Geometry check sheet. Reference: the model listing, model coordinates, mm. Face numbers are marked on the shaded views. A direction names the side the tool comes from. Coordinates: 2 decimals unless noted, no trailing zeros. Write each loop counter-clockwise with the first axis right and the second up, starting at its lowest first coordinate (ties: lowest second). Pieces come first, ordered by that corner, then holes.
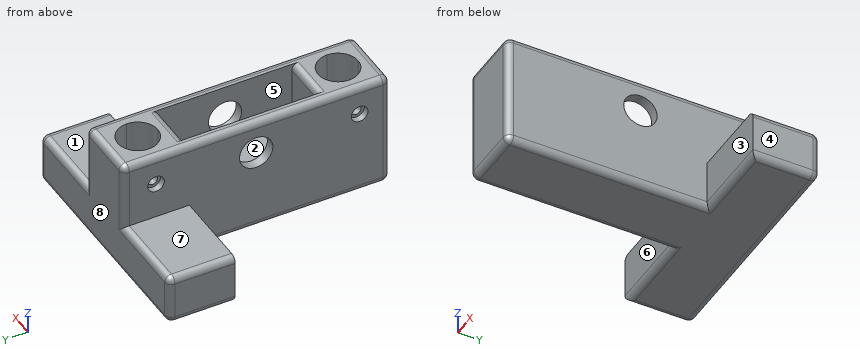
from build123d import *

# Parameters (mm, degrees)
F1_DEPTH        = 15
F2_W            = 20
F2_H            = 20
F3_DEPTH        = 20
F5_DEPTH        = 15
F6_W            = 20
F6_H            = 20
F7_DEPTH        = 20
F9_DEPTH        = 15
F10_W           = 3
F10_H           = 40
F11_DEPTH       = 20
F12_R           = 5
F13_DEPTH       = 25
F14_R           = 2
F15_R           = 2
F16_R           = 2
F17_R           = 2
F19_D           = 3.1
F19_DEPTH       = 6
F19_CBORE_D     = 5
F19_CBORE_DEPTH = 2


with BuildPart() as f1:
    # F0 (on Top) → F1 (new body)
    with BuildSketch(Plane.XY):
        Polygon((-20, 0), (0, 0), (0, 60), (25, 60), (25, 80), (-45, 80), (-45, 60), (-20, 60), align=None)
    extrude(amount=F1_DEPTH)

    # F2 (on face) → F3 (join)
    with BuildSketch(Plane.XY.offset(15)):
        with Locations((-10, 10)):
            Rectangle(F2_W, F2_H)
    extrude(amount=F3_DEPTH)

    # F4 (on face) → F5 (cut)
    with BuildSketch(Plane.XY.offset(35)):
        with BuildLine():
            ThreePointArc((-10, 4), (-5.757359, 5.757359), (-4, 10))
            ThreePointArc((-4, 10), (-14.242641, 14.242641), (-10, 4))
        make_face()
    extrude(amount=-F5_DEPTH, mode=Mode.SUBTRACT)

    # F6 (on face) → F7 (join)
    with BuildSketch(Plane.XY.offset(15)):
        with Locations((-10, 70)):
            Rectangle(F6_W, F6_H)
    extrude(amount=F7_DEPTH)

    # F8 (on face) → F9 (cut)
    with BuildSketch(Plane.XY.offset(35)):
        with BuildLine():
            ThreePointArc((-10, 64), (-5.757359, 65.757359), (-4, 70))
            ThreePointArc((-4, 70), (-14.242641, 74.242641), (-10, 64))
        make_face()
    extrude(amount=-F9_DEPTH, mode=Mode.SUBTRACT)

    # F10 (on face) → F11 (join)
    with BuildSketch(Plane.XY.offset(15)):
        with Locations((-1.5, 40)):
            Rectangle(F10_W, F10_H)
        with Locations((-18.5, 40)):
            Rectangle(F10_W, F10_H)
    extrude(amount=F11_DEPTH)

    # F12 (on face) → F13 (cut)
    with BuildSketch(Plane(origin=(-20, 0, 0), x_dir=(0, -1, 0), z_dir=(-1, 0, 0))):
        with Locations((-40, 25)):
            Circle(F12_R)
    extrude(amount=-F13_DEPTH, mode=Mode.SUBTRACT)

    # F14
    f14_edges = [f1.edges().sort_by_distance(p)[0] for p in [
        (-20, 40, 35),
        (0, 40, 35),
    ]]
    fillet(f14_edges, radius=F14_R)

    # F15
    f15_edges = [f1.edges().sort_by_distance(p)[0] for p in [
        (-10, 20, 35),
        (-10, 60, 35),
        (-10, 80, 35),
        (-10, 0, 35),
    ]]
    fillet(f15_edges, radius=F15_R)

    # F16
    f16_edges = [f1.edges().sort_by_distance(p)[0] for p in [
        (-1, 80, 15),
        (12.5, 80, 15),
        (-19, 80, 15),
        (-32.5, 80, 15),
    ]]
    fillet(f16_edges, radius=F16_R)

    # F17
    f17_edges = [f1.edges().sort_by_distance(p)[0] for p in [
        (-20, 31, 0),
        (-32.5, 60, 0),
        (12.5, 60, 0),
        (-45, 70, 0),
        (25, 70, 0),
        (-10, 80, 0),
        (-45, 80, 6.5),
        (25, 80, 6.5),
    ]]
    fillet(f17_edges, radius=F17_R)

    # F19
    with Locations(Plane(origin=(-20, 0, 0), x_dir=(0, -1, 0), z_dir=(-1, 0, 0))):
        with Locations((-70, 26), (-9, 26)):
            CounterBoreHole(F19_D / 2, F19_CBORE_D / 2, F19_CBORE_DEPTH, depth=F19_DEPTH)


solid = f1.part
1. Sectioned sample at A-A, the plane y = 40. Record the boundary of the cut face in (x, z), and give its area (3 significant figures).
Computed values:
outline: (-20, 2) arc R2 ccw to (-18, 0) - (-2, 0) arc R2 ccw to (0, 2) - (0, 20) - (-3, 20) - (-3, 15) - (-17, 15) - (-17, 20) - (-20, 20) - close; (-20, 30) - (-17, 30) - (-17, 35) - (-18, 35) arc R2 ccw to (-20, 33) - close; (-3, 30) - (0, 30) - (0, 33) arc R2 ccw to (-2, 35) - (-3, 35) - close
area: 357 mm2
2. Sectioned sample at B-B, the plane z = 9. Record the boundary of the cut face in (x, y).
Computed values:
outline: (-45, 60) - (-20, 60) - (-20, 2) arc R2 ccw to (-18, 0) - (-2, 0) arc R2 ccw to (0, 2) - (0, 60) - (25, 60) - (25, 78) arc R2 ccw to (23, 80) - (-43, 80) arc R2 ccw to (-45, 78) - close
3. Sectioned sample at D-D, the plane y = 51. Record the boundary of the cut face in (x, z).
Computed values:
outline: (-20, 2) arc R2 ccw to (-18, 0) - (-2, 0) arc R2 ccw to (0, 2) - (0, 33) arc R2 ccw to (-2, 35) - (-3, 35) - (-3, 15) - (-17, 15) - (-17, 35) - (-18, 35) arc R2 ccw to (-20, 33) - close
4. Draft check along Y on the marked faces 5, 6, 7 and 8. Enter one of: released by +Y, released by -Y, zero draft, split by the parting line, or undercut.
Computed values:
face 5: undercut
face 6: released by -Y
face 7: zero draft
face 8: released by +Y
5. Sectioned sample at C-C, the plane x = -41. Record the boundary of the cut face in (y, z).
Computed values:
outline: (60, 2) arc R2 ccw to (62, 0) - (78, 0) arc R2 ccw to (80, 2) - (80, 13) arc R2 ccw to (78, 15) - (60, 15) - close
6. Thickness scan on line 1 along Y through (x, z) = (-16.8, 26); line 2 along Z through (x, y) = (-16.5, 70); line 3 along X through (y, z) = (56, 24). Record the ranges inside material, lowest first.
Computed values:
line 1: y = 0 to 7.45, 10.55 to 20, 60 to 68.45, 71.55 to 80
line 2: z = 0 to 24.45, 27.55 to 35
line 3: x = -20 to -17, -3 to 0
7. Access from +Z, -Z, +X, -X, +Y, -Y to the whole of each face (thin tool, end or side, straight path). Record for the marked faces 1, 2, 3 and 4.
Computed values:
face 1: +Z, +X, +Y, -Y
face 2: +Z
face 3: +Z, -Z, +X, -Y
face 4: +Z, -Z, +X, +Y, -Y
8. Gauge pin test, flat ends, axial feed: pin 1 Ø8 at (y, z) = (15, 9) entering from -X; pin 2 Ø6 at (x, z) = (5, 13.5) entering from -Y; pin 3 Ø14.5 at (x, z) = (6.5, 8) entering from -Y; pin 4 Ø6 at (y, z) = (40, 25) entering from -X. Record the tip position at first contact, or that the pin passes through.
Computed values:
pin 1: stops at x = -20
pin 2: stops at y = 60
pin 3: stops at y = 0.44
pin 4: passes through
